Design review of the part built by this model. Coordinates are the model's own, in mm. Coordinates: 2 decimals unless noted, no trailing zeros. Loops run counter-clockwise (first coordinate to the right, second up) from the corner with the lowest first, then second, coordinate; pieces in that order, holes last. Notation, with made-up numbers: (38.25, 0) -> (67.25, 0) arc R15 ccw to (67.25, 20) -> close; hole circle Ø7 at (63.25, 14). An arc over 180 degrees is marked (long way). Use a Markdown table: item, result. Add a question column.
Q1. Clearance check with flat-ended pins moving along their axes: pin 1 Ø3 at (y, z) = (180.5, 4.5) entering from -X; pin 2 Ø1 at (x, z) = (72, 3.5) entering from -Y; pin 3 Ø5 at (x, z) = (-5.5, 7.5) entering from -Y. State where each tip first meets the part, or that it passes through.
Q2. Take a section at D-D on y = 361.5. Write out the cut boundary in (x, z), plus the area to 3 significant figures.
Q3. For probe 1 along Y at (x, z) = (52.5, 2.5); probe 2 along X at (y, z) = (127, 4.75); probe 3 along Y at (x, z) = (20, 1.25), list the stretches that pass through material, from the lowest coordinate up.
Q4. Take a section at A-A on y = 158.5. Write out the cut boundary in (x, z).
Q5. Take a section at C-C on x = 160. Write out the cut boundary in (y, z), plus the area to 3 significant figures.
Q6. Take a section at B-B on z = 2. Write out the cut boundary in (x, y).
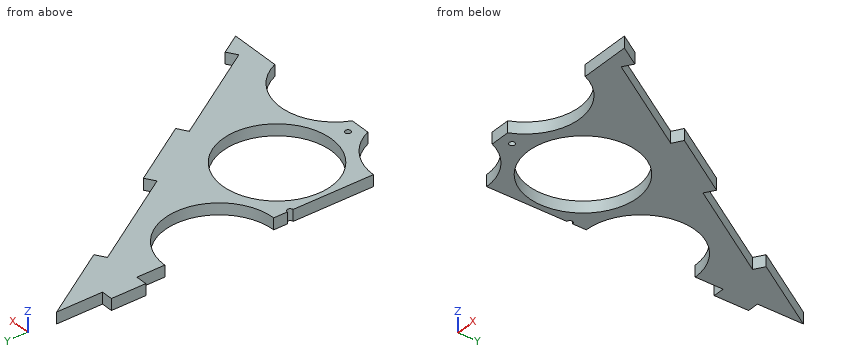
from build123d import *

# Parameters (mm, degrees)
ESQUISSE1_R             = 47.5
BOSS_EXTRU_1_DEPTH      = 10
ESQUISSE3_W             = 100
ESQUISSE3_H             = 10
ENL_V_MAT_EXTRU_1_DEPTH = 11
ESQUISSE4_R             = 2.5
ENL_V_MAT_EXTRU_2_DEPTH = 11
ESQUISSE6_W             = 150
ESQUISSE6_H             = 120
BOSS_EXTRU_2_DEPTH      = 10
ESQUISSE7_W             = 10
ESQUISSE7_H             = 50
ESQUISSE7_W_2           = 50
ESQUISSE7_H_2           = 9.570800355
ENL_V_MAT_EXTRU_3_DEPTH = 10
ENL_V_MAT_EXTRU_5_DEPTH = 10
ESQUISSE11_W            = 10
ESQUISSE11_H            = 30
BOSS_EXTRU_4_DEPTH      = 10


with BuildPart() as part:
    # Esquisse1 → Boss.-Extru.1 (new body)
    with BuildSketch(Plane.XY):
        Polygon((-310, -75.642859016), (0, 414.561180135), (310, -75.642859016), align=None)
        with Locations((-157.5, 0)):
            Circle(ESQUISSE1_R, mode=Mode.SUBTRACT)
        with Locations((-52.5, 0)):
            Circle(ESQUISSE1_R, mode=Mode.SUBTRACT)
        with Locations((52.5, 0)):
            Circle(ESQUISSE1_R, mode=Mode.SUBTRACT)
        with Locations((157.5, 0)):
            Circle(ESQUISSE1_R, mode=Mode.SUBTRACT)
        with Locations((-105, 90.932667397)):
            Circle(ESQUISSE1_R, mode=Mode.SUBTRACT)
        with Locations((0, 90.932667397)):
            Circle(ESQUISSE1_R, mode=Mode.SUBTRACT)
        with Locations((105, 90.932667397)):
            Circle(ESQUISSE1_R, mode=Mode.SUBTRACT)
        with Locations((-52.5, 181.865334795)):
            Circle(ESQUISSE1_R, mode=Mode.SUBTRACT)
        with Locations((52.5, 181.865334795)):
            Circle(ESQUISSE1_R, mode=Mode.SUBTRACT)
        with Locations((0, 272.798002192)):
            Circle(ESQUISSE1_R, mode=Mode.SUBTRACT)
    extrude(amount=BOSS_EXTRU_1_DEPTH)

    # Esquisse3 → Enlèv. mat.-Extru.1 (cut, through all)
    with BuildSketch(Plane.XY.offset(10)):
        Polygon((-269.913793103, -12.254405678), (-261.461999325, -17.599233264), (-208.013723463, 66.918704521), (-216.465517241, 72.263532107), align=None)
        Polygon((-181.724137931, 127.200191667), (-173.272344153, 121.855364081), (-119.82406829, 206.373301865), (-128.275862069, 211.718129452), align=None)
        Polygon((-93.534482759, 266.654789012), (-85.08268898, 261.309961425), (-31.634413118, 345.82789921), (-40.086206897, 351.172726796), align=None)
        Polygon((269.913793103, -12.254405678), (261.461999325, -17.599233264), (208.013723463, 66.918704521), (216.465517241, 72.263532107), align=None)
        Polygon((181.724137931, 127.200191667), (173.272344153, 121.855364081), (119.82406829, 206.373301865), (128.275862069, 211.718129452), align=None)
        Polygon((93.534482759, 266.654789012), (85.08268898, 261.309961425), (31.634413118, 345.82789921), (40.086206897, 351.172726796), align=None)
        with Locations((-160, -70.642859016)):
            Rectangle(ESQUISSE3_W, ESQUISSE3_H)
        with Locations((160, -70.642859016)):
            Rectangle(ESQUISSE3_W, ESQUISSE3_H)
    extrude(amount=-ENL_V_MAT_EXTRU_1_DEPTH, mode=Mode.SUBTRACT)

    # Esquisse4 → Enlèv. mat.-Extru.2 (cut, through all)
    with BuildSketch(Plane.XY.offset(10)):
        with Locations((-157.5, -55.642859016)):
            Circle(ESQUISSE4_R)
        with Locations((-52.5, -55.642859016)):
            Circle(ESQUISSE4_R)
        with Locations((52.5, -55.642859016)):
            Circle(ESQUISSE4_R)
        with Locations((157.5, -55.642859016)):
            Circle(ESQUISSE4_R)
        with Locations((-105, 29.047375097)):
            Circle(ESQUISSE4_R)
        with Locations((0, 29.047375097)):
            Circle(ESQUISSE4_R)
        with Locations((105, 29.047375097)):
            Circle(ESQUISSE4_R)
        with Locations((-52.5, 119.980042494)):
            Circle(ESQUISSE4_R)
        with Locations((52.5, 119.980042494)):
            Circle(ESQUISSE4_R)
        with Locations((0, 210.912709891)):
            Circle(ESQUISSE4_R)
    extrude(amount=-ENL_V_MAT_EXTRU_2_DEPTH, mode=Mode.SUBTRACT)

    # Esquisse6 → Boss.-Extru.2 (add)
    with BuildSketch(Plane.XY.offset(10)):
        with Locations((0, -135.642859016)):
            Rectangle(ESQUISSE6_W, ESQUISSE6_H)
    extrude(amount=-BOSS_EXTRU_2_DEPTH)

    # Esquisse7 → Enlèv. mat.-Extru.3 (cut)
    with BuildSketch(Plane.XY.offset(10)):
        with Locations((-70, -135.642859016)):
            Rectangle(ESQUISSE7_W, ESQUISSE7_H)
        with Locations((0, -190.857458839)):
            Rectangle(ESQUISSE7_W_2, ESQUISSE7_H_2)
        with Locations((70, -135.642859016)):
            Rectangle(ESQUISSE7_W, ESQUISSE7_H)
    extrude(amount=-ENL_V_MAT_EXTRU_3_DEPTH, mode=Mode.SUBTRACT)

    # Esquisse10 → Enlèv. mat.-Extru.5 (cut)
    with BuildSketch(Plane.XY.offset(10)):
        Polygon((0, 414.561180135), (0, 109.461180135), (337.106568203, 109.461180135), (337.106568203, -228.052583807), (-388.969117157, -228.052583807), (-388.969117157, 414.561180135), align=None)
    extrude(amount=-ENL_V_MAT_EXTRU_5_DEPTH, mode=Mode.SUBTRACT)

    # Esquisse11 → Boss.-Extru.4 (add)
    with BuildSketch(Plane.XY.offset(10)):
        with Locations((-5, 359.561180135)):
            Rectangle(ESQUISSE11_W, ESQUISSE11_H)
    extrude(amount=-BOSS_EXTRU_4_DEPTH)


solid = part.part
Answer list:
| question | item | result |
|---|---|---|
| 1 | pin 1 | x = 0 |
| 1 | pin 2 | y = 124.61 |
| 1 | pin 3 | y = 344.56 |
| 2 | outline | (-10, 0) -> (33.56, 0) -> (33.56, 10) -> (-10, 10) -> close |
| 2 | area | 436 mm² |
| 3 | probe 1 | 109.46 to 117.48, 122.48 to 134.37, 229.37 to 312.83 |
| 3 | probe 2 | 30.91 to 74.09, 135.91 to 170.02, 181.41 to 181.85 |
| 3 | probe 3 | 134.02 to 147.22, 216.51 to 229.71, 315.88 to 382.94 |
| 4 | outline | (0, 0) -> (11.14, 0) -> (11.14, 10) -> (0, 10) -> close; (93.86, 0) -> (150.1, 0) -> (150.1, 10) -> (93.86, 10) -> close |
| 5 | outline | (109.46, 0) -> (142.84, 0) -> (142.84, 10) -> (109.46, 10) -> close |
| 5 | area | 334 mm² |
| 6 | outline | (-10, 344.56) -> (0, 344.56) -> (0, 320.3) arc R47.5 cw to (0, 225.3) -> (0, 213.41) arc R2.5 cw to (0, 208.41) -> (0, 138.43) arc R47.5 cw to (43.74, 109.46) -> (61.26, 109.46) arc R47.5 cw to (148.74, 109.46) -> (192.94, 109.46) -> (181.72, 127.2) -> (173.27, 121.86) -> (119.82, 206.37) -> (128.28, 211.72) -> (93.53, 266.65) -> (85.08, 261.31) -> (31.63, 345.83) -> (40.09, 351.17) -> (0, 414.56) -> (0, 374.56) -> (-10, 374.56) -> close; hole circle Ø95 at (52.5, 181.87); hole circle Ø5 at (52.5, 119.98) |
